Can you work these out from the model? Positions are in its coordinate system, mm. A direction names the side the tool comes from. Give positions to 0.01 mm unless a question says otherwise; leave off trailing zeros. Order: outer loops, then holes, each group sorted by start corner. A loop starts at its lowest first (then second) coordinate and runs counter-clockwise, first axis right, second up.
```python
from build123d import *

# Parameters (mm, degrees)
SKETCH1_R           = 14.2875
SKETCH1_R_2         = 1.6002
SKETCH1_R_3         = 2.4892
BOSS_EXTRUDE3_DEPTH = 3.175
SKETCH2_W           = 355.6
SKETCH2_H           = 19.05
CUT_EXTRUDE1_DEPTH  = 290.621961572
FILLET1_R           = 19.05


with BuildPart() as part:
    # Sketch1 → Boss-Extrude3 (new body)
    with BuildSketch(Plane.XY):
        with BuildLine():
            Line((120.65, -152.4), (120.65, -6.35))
            Line((120.65, -6.35), (120.65, 6.35))
            ThreePointArc((120.65, 6.35), (124.369743879, 15.330256121), (133.35, 19.05))
            Line((133.35, 19.05), (165.1, 19.05))
            ThreePointArc((165.1, 19.05), (174.080256121, 15.330256121), (177.8, 6.35))
            Line((177.8, 6.35), (177.8, -6.35))
            Line((177.8, -6.35), (177.8, -222.25))
            ThreePointArc((177.8, -222.25), (175.940128061, -226.740128061), (171.45, -228.6))
            Line((171.45, -228.6), (12.7, -228.6))
            Line((12.7, -228.6), (-12.7, -228.6))
            Line((-12.7, -228.6), (-171.45, -228.6))
            ThreePointArc((-171.45, -228.6), (-175.940128061, -226.740128061), (-177.8, -222.25))
            Line((-177.8, -222.25), (-177.8, -6.35))
            Line((-177.8, -6.35), (-177.8, 6.35))
            ThreePointArc((-177.8, 6.35), (-174.080256121, 15.330256121), (-165.1, 19.05))
            Line((-165.1, 19.05), (-133.35, 19.05))
            ThreePointArc((-133.35, 19.05), (-124.369743879, 15.330256121), (-120.65, 6.35))
            Line((-120.65, 6.35), (-120.65, -6.35))
            Line((-120.65, -6.35), (-120.65, -152.4))
            ThreePointArc((-120.65, -152.4), (-113.210512242, -170.360512242), (-95.25, -177.8))
            Line((-95.25, -177.8), (-12.7, -177.8))
            Line((-12.7, -177.8), (12.7, -177.8))
            Line((12.7, -177.8), (95.25, -177.8))
            ThreePointArc((95.25, -177.8), (113.210512242, -170.360512242), (120.65, -152.4))
        make_face()
        with Locations((141.605, -25.4)):
            Circle(SKETCH1_R, mode=Mode.SUBTRACT)
        with Locations(Location((-141.605, -25.4, 0), (0, 0, 180))):
            Circle(SKETCH1_R, mode=Mode.SUBTRACT)
        with Locations((-141.605, -203.2)):
            Circle(SKETCH1_R, mode=Mode.SUBTRACT)
        with Locations((-141.605, -184.722481985)):
            Circle(SKETCH1_R_2, mode=Mode.SUBTRACT)
        with Locations((-125.603, -193.961240992)):
            Circle(SKETCH1_R_2, mode=Mode.SUBTRACT)
        with Locations((-125.603, -212.438759008)):
            Circle(SKETCH1_R_2, mode=Mode.SUBTRACT)
        with Locations((-141.605, -221.677518015)):
            Circle(SKETCH1_R_2, mode=Mode.SUBTRACT)
        with Locations((-157.607, -212.438759008)):
            Circle(SKETCH1_R_2, mode=Mode.SUBTRACT)
        with Locations((-157.607, -193.961240992)):
            Circle(SKETCH1_R_2, mode=Mode.SUBTRACT)
        with Locations(Location((157.607, -212.438759008, 0), (0, 0, 180))):
            Circle(SKETCH1_R_2, mode=Mode.SUBTRACT)
        with Locations(Location((157.607, -193.961240992, 0), (0, 0, 180))):
            Circle(SKETCH1_R_2, mode=Mode.SUBTRACT)
        with Locations(Location((141.605, -184.722481985, 0), (0, 0, 180))):
            Circle(SKETCH1_R_2, mode=Mode.SUBTRACT)
        with Locations(Location((125.603, -193.961240992, 0), (0, 0, 180))):
            Circle(SKETCH1_R_2, mode=Mode.SUBTRACT)
        with Locations(Location((125.603, -212.438759008, 0), (0, 0, 180))):
            Circle(SKETCH1_R_2, mode=Mode.SUBTRACT)
        with Locations(Location((141.605, -221.677518015, 0), (0, 0, 180))):
            Circle(SKETCH1_R_2, mode=Mode.SUBTRACT)
        with Locations(Location((141.605, -203.2, 0), (0, 0, 180))):
            Circle(SKETCH1_R, mode=Mode.SUBTRACT)
        with Locations((-76.2, -203.2)):
            Circle(SKETCH1_R_3, mode=Mode.SUBTRACT)
        with Locations(Location((76.2, -203.2, 0), (0, 0, 180))):
            Circle(SKETCH1_R_3, mode=Mode.SUBTRACT)
        with Locations((-25.4, -203.2)):
            Circle(SKETCH1_R_3, mode=Mode.SUBTRACT)
        with Locations((-127, -171.45)):
            Circle(SKETCH1_R_3, mode=Mode.SUBTRACT)
        with Locations((-149.225, 6.35)):
            Circle(SKETCH1_R_3, mode=Mode.SUBTRACT)
        with Locations(Location((127, -171.45, 0), (0, 0, 180))):
            Circle(SKETCH1_R_3, mode=Mode.SUBTRACT)
        with Locations(Location((149.225, 6.35, 0), (0, 0, 180))):
            Circle(SKETCH1_R_3, mode=Mode.SUBTRACT)
        with Locations((-168.275, -209.55)):
            Circle(SKETCH1_R_3, mode=Mode.SUBTRACT)
        with Locations(Location((168.275, -209.55, 0), (0, 0, 180))):
            Circle(SKETCH1_R_3, mode=Mode.SUBTRACT)
        with Locations((-165.1, -76.2)):
            Circle(SKETCH1_R_3, mode=Mode.SUBTRACT)
        with Locations(Location((165.1, -76.2, 0), (0, 0, 180))):
            Circle(SKETCH1_R_3, mode=Mode.SUBTRACT)
        with Locations(Location((25.4, -203.2, 0), (0, 0, 180))):
            Circle(SKETCH1_R_3, mode=Mode.SUBTRACT)
    extrude(amount=BOSS_EXTRUDE3_DEPTH)

    # Sketch2 → Cut-Extrude1 (cut, through all)
    with BuildSketch(Plane.XY.offset(3.175)):
        with Locations((0, 9.525)):
            Rectangle(SKETCH2_W, SKETCH2_H)
    extrude(amount=-CUT_EXTRUDE1_DEPTH, mode=Mode.SUBTRACT)

    # Fillet1
    fillet1_edges = [part.edges().sort_by_distance(p)[0] for p in [
        (-177.8, 0, 1.5875),
        (120.65, 0, 1.5875),
        (177.8, 0, 1.5875),
        (-120.65, 0, 1.5875),
    ]]
    fillet(fillet1_edges, radius=FILLET1_R)


solid = part.part
```
1) If I drill on line 1 (Y direction, x = 141.5, z = 2.1); line 2 (X direction, y = -144, z = 2.8), over which ranges is the centre line in solid material (lowest first)?
2) Suppose I cut it at B-B (y = -56). Please give me the cut outline in (x, z) (3 decimals), and give its area (3 significant figures).
3) Which directions (+Z, -Z, +X, -X, +Y, -Y) give clear straight access to the entire face, cutting with the end or side of a thin tool? Please do faces 1 (the face through (155.88, -203.83, 1.57)), 2 (the face through (113.01, -170.56, 1.57)).
4) Suppose I cut it at A-A (y = -25.4). Give the number of separate pieces and of enclosed holes in the cut face, and give its area (3 significant figures).
5) We'd pull the mould along X, two halves only. Please class faces 3 (the face through (172.07, -5.43, 1.57)), 4 (the face through (131.075, -15.744, 1.565)), 5 (the face through (126.08, -5.73, 1.61)), 6 (the face through (-172.07, -5.43, 1.57)): +X half, -X half, draft (parallel to the pull), parting line (faces both ways), or undercut.
6) Suppose I cut it at C-C (x = -34). Please give me the cut outline in (y, z) (3 decimals).
Results:
1. line 1: y = -228.6 to -223.27, -220.08 to -217.49, -188.91 to -186.32, -183.13 to -39.69, -11.11 to 0
1. line 2: x = -177.8 to -120.65, 120.65 to 177.8
2. outline: (-177.8, 0) - (-120.65, 0) - (-120.65, 3.175) - (-177.8, 3.175) - close; (120.65, 0) - (177.8, 0) - (177.8, 3.175) - (120.65, 3.175) - close
2. area: 363 mm2
3. face 1: +Z, -Z
3. face 2: +Z, -Z, +Y
4. separate pieces: 4
4. enclosed holes: 0
4. area: 181 mm2
5. face 3: +X half
5. face 4: undercut
5. face 5: undercut
5. face 6: -X half
6. outline: (-228.6, 0) - (-177.8, 0) - (-177.8, 3.175) - (-228.6, 3.175) - close
